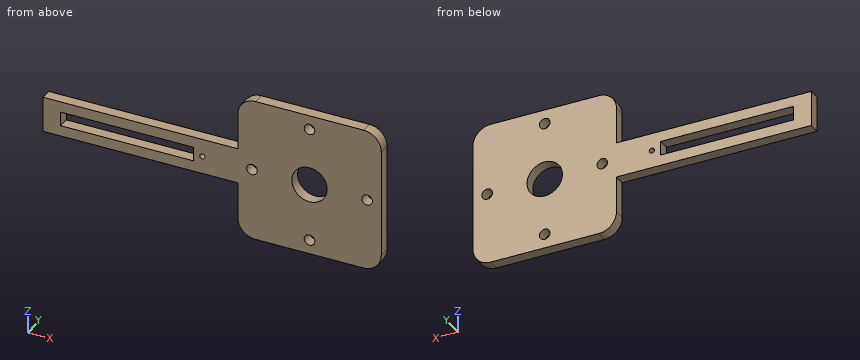
from build123d import *

# Parameters (mm, degrees)
SKETCH1_R           = 10
SKETCH1_R_2         = 3
SKETCH1_R_3         = 1.5
SKETCH1_W           = 75
SKETCH1_H           = 8
BOSS_EXTRUDE1_DEPTH = 6.35
FILLET1_R           = 10


with BuildPart() as part:
    # Sketch1 → Boss-Extrude1 (new body)
    with BuildSketch(Plane(origin=(0, 0, 0), x_dir=(1, 0, 0), z_dir=(0, 1, 0))):
        Polygon((-40.5, 40.5), (40.5, 40.5), (40.5, -40.5), (-40.5, -40.5), (-40.5, -10), (-140.5, -10), (-150.5, -10), (-150.5, 10), (-140.5, 10), (-40.5, 10), align=None)
        with Locations(Location((0, 0, 0), (0, 0, 270))):
            Circle(SKETCH1_R, mode=Mode.SUBTRACT)
        with Locations(Location((0, 32.5, 0), (0, 0, 270))):
            Circle(SKETCH1_R_2, mode=Mode.SUBTRACT)
        with Locations(Location((-32.5, 0, 0), (0, 0, 270))):
            Circle(SKETCH1_R_2, mode=Mode.SUBTRACT)
        with Locations(Location((0, -32.5, 0), (0, 0, 270))):
            Circle(SKETCH1_R_2, mode=Mode.SUBTRACT)
        with Locations(Location((32.5, 0, 0), (0, 0, 270))):
            Circle(SKETCH1_R_2, mode=Mode.SUBTRACT)
        with Locations(Location((-60.5, 0, 0), (0, 0, 270))):
            Circle(SKETCH1_R_3, mode=Mode.SUBTRACT)
        with Locations((-103, 0)):
            Rectangle(SKETCH1_W, SKETCH1_H, mode=Mode.SUBTRACT)
    extrude(amount=BOSS_EXTRUDE1_DEPTH)

    # Fillet1
    fillet1_edges = [part.edges().sort_by_distance(p)[0] for p in [
        (40.5, 3.175, 40.5),
        (-40.5, 3.175, 40.5),
        (-40.5, 3.175, -40.5),
        (40.5, 3.175, -40.5),
    ]]
    fillet(fillet1_edges, radius=FILLET1_R)


solid = part.part
Read the model definition and answer for the solid it produces. Units are mm, in the model's axes. Round coordinates to 2 decimals unless told otherwise and drop trailing zeros. Write each loop counter-clockwise with the first axis right and the second up, starting at its lowest first coordinate (ties: lowest second). Pieces come first, ordered by that corner, then holes. Notation, with made-up numbers: M -23.75,45 L 28.25,45 A28 ccw 28.25,72 Z; hole C -39.75,44 d11. An arc over 180 degrees is marked long. Use a Markdown table: item, result.
1) The part is cut by section D-D (z = 32.5). Write down the section's boundary in (x, y), plus the area to 3 significant figures.
Answers follow:
| item | result |
|---|---|
| outline | M -40.3,0 L -3,0 L -3,6.35 L -40.3,6.35 Z; M 3,0 L 40.3,0 L 40.3,6.35 L 3,6.35 Z |
| area | 474 mm2 |
2) Straight lines are drawn through the part: line 1 along X through (y, z) = (2, 0); line 2 along Z through (x, y) = (-84, 2.75); line 3 along Z through (x, y) = (-1, 3.75). For each, find the intervals that lie inside material, in ascending order. Write a range as [from, to].
Answers follow:
| item | result |
|---|---|
| line 1 | x = [-150.5, -140.5], [-65.5, -62], [-59, -35.5], [-29.5, -10], [10, 29.5], [35.5, 40.5] |
| line 2 | z = [-10, -4], [4, 10] |
| line 3 | z = [-40.5, -35.33], [-29.67, -9.95], [9.95, 29.67], [35.33, 40.5] |
3) The part is cut by section B-B (x = -76). Write down the section's boundary in (y, z), plus the area to 3 significant figures.
Answers follow:
| item | result |
|---|---|
| outline | M 0,-10 L 6.35,-10 L 6.35,-4 L 0,-4 Z; M 0,4 L 6.35,4 L 6.35,10 L 0,10 Z |
| area | 76.2 mm2 |
4) Flat-ended cylindrical pins translate along their axes: pin 1 (12 mm diameter, centred on x = 0, z = 0, fed in from -Y); pin 2 (7 mm diameter, centred on x = 0, z = 32.5, fed in from +Y); pin 3 (3 mm diameter, centred on x = -107, y = 3.5, fed in from -Z); pin 4 (1.9 mm diameter, centred on x = -87, y = 4.5, fed in from +Z). Find the tip coordinate at first contact, or state that the pin passes through.
Answers follow:
| item | result |
|---|---|
| pin 1 | passes through |
| pin 2 | stops at y = 6.35 |
| pin 3 | stops at z = -10 |
| pin 4 | stops at z = 10 |
5) The part is cut by section C-C (y = 2.75). Write down the section's boundary in (x, z).
Answers follow:
| item | result |
|---|---|
| outline | M -150.5,-10 L -40.5,-10 L -40.5,-30.5 A10 ccw -30.5,-40.5 L 30.5,-40.5 A10 ccw 40.5,-30.5 L 40.5,30.5 A10 ccw 30.5,40.5 L -30.5,40.5 A10 ccw -40.5,30.5 L -40.5,10 L -150.5,10 Z; hole M -140.5,-4 L -65.5,-4 L -65.5,4 L -140.5,4 Z; hole C -60.5,0 d3; hole C -32.5,0 d6; hole C 0,0 d20; hole C 0,-32.5 d6; hole C 0,32.5 d6; hole C 32.5,0 d6 |
6) The part is cut by section A-A (x = 0). Write down the section's boundary in (y, z).
Answers follow:
| item | result |
|---|---|
| outline | M 0,-40.5 L 6.35,-40.5 L 6.35,-35.5 L 0,-35.5 Z; M 0,-29.5 L 6.35,-29.5 L 6.35,-10 L 0,-10 Z; M 0,10 L 6.35,10 L 6.35,29.5 L 0,29.5 Z; M 0,35.5 L 6.35,35.5 L 6.35,40.5 L 0,40.5 Z |
